Design review of the part built by this model. Coordinates are the model's own, in mm. Coordinates: 2 decimals unless noted, no trailing zeros. Loops run counter-clockwise (first coordinate to the right, second up) from the corner with the lowest first, then second, coordinate; pieces in that order, holes last. Notation, with made-up numbers: M 2,45 L 38,45 A28 ccw 38,78 Z; hole C -27,25.5 d3. An arc over 180 degrees is marked long. Answer as a JSON object with one key per item and string values. Group by question number.
1. Consider section A-A (x = 84.5). State the section outline as (y, z) points, then the cut area to 3 significant figures.
2. Consider section B-B (z = 0.4). Count the separate pieces of the cut face and the enclosed holes in it, then the cut area to 3 significant figures.
3. To check wall thickness, follow probe 1 along X at (y, z) = (-30.5, 0.2); probe 2 along Y at (x, z) = (-32.5, 1.5) (3 decimals); probe 3 along Y at (x, z) = (-54.5, 1.85). State the ranges of each line that lie inside material, in increasing order.
4. Insertion check: pin 1 (0.6 mm diameter, centred on x = -33.5, z = 1, fed in from +Y) (3 decimals). The pin has a flat end and moves straight along its axis. Give the tip position at first contact, or say it passes through.
from build123d import *

# Parameters (mm, degrees)
SKETCH_1_R          = 2.05
SKETCH_1_R_2        = 4
SKETCH_1_R_3        = 2.332988974
SKETCH_1_R_4        = 1.601067765
SKETCH_1_W          = 8.8
SKETCH_1_H          = 2.8
SKETCH_1_W_2        = 2.5
SKETCH_1_H_2        = 8.5
SKETCH_1_W_3        = 8.5
SKETCH_1_H_3        = 2.5
SKETCH_1_W_4        = 241.301375666
SKETCH_1_H_4        = 241.301375666
SKETCH_1_W_5        = 2.3
SKETCH_1_H_5        = 4.3
EXTRUDE_1_DEPTH     = 2
SKETCH_2_W          = 15.371335927
SKETCH_2_H          = 8.514117998
SKETCH_2_W_2        = 8.829080761
SKETCH_2_H_2        = 8.5
SKETCH_2_W_3        = 10.335603127
SKETCH_2_W_4        = 8.5
SKETCH_2_H_3        = 5.29768324
SKETCH_2_H_4        = 6.445558592
SKETCH_2_H_5        = 5.884818728
CUT_EXTRUDE_1_DEPTH = 2
FILLET_1_R          = 2


with BuildPart() as part:
    # 草图1 → 凸台-拉伸1 (new body)
    with BuildSketch(Plane.XY):
        Polygon((-150.650687833, -150.650687833), (-150.650687833, 150.650687833), (150.650687833, 150.650687833), (200.650687833, 150.650687833), (200.650687833, -278.650687833), (150.650687833, -278.650687833), (-150.650687833, -278.650687833), align=None)
        with Locations((0.724285714, -142.895)):
            Circle(SKETCH_1_R, mode=Mode.SUBTRACT)
        with Locations((66.724285714, -142.895)):
            Circle(SKETCH_1_R, mode=Mode.SUBTRACT)
        with Locations((-65.275714286, -142.895)):
            Circle(SKETCH_1_R, mode=Mode.SUBTRACT)
        with Locations((-143.125714286, 66.955)):
            Circle(SKETCH_1_R, mode=Mode.SUBTRACT)
        with Locations((-143.125714286, 0.955)):
            Circle(SKETCH_1_R, mode=Mode.SUBTRACT)
        with Locations((-143.125714286, -65.045)):
            Circle(SKETCH_1_R, mode=Mode.SUBTRACT)
        with Locations((66.874285714, 144.955)):
            Circle(SKETCH_1_R, mode=Mode.SUBTRACT)
        with Locations((0.874285714, 144.955)):
            Circle(SKETCH_1_R, mode=Mode.SUBTRACT)
        with Locations((-65.125714286, 144.955)):
            Circle(SKETCH_1_R, mode=Mode.SUBTRACT)
        with Locations((144.874285714, -65.045)):
            Circle(SKETCH_1_R, mode=Mode.SUBTRACT)
        with Locations((144.874285714, 0.955)):
            Circle(SKETCH_1_R, mode=Mode.SUBTRACT)
        with Locations((144.874285714, 66.955)):
            Circle(SKETCH_1_R, mode=Mode.SUBTRACT)
        with Locations((-130.650687833, -130.650687833)):
            Circle(SKETCH_1_R_2, mode=Mode.SUBTRACT)
        with Locations((-130.650687833, 130.650687833)):
            Circle(SKETCH_1_R_2, mode=Mode.SUBTRACT)
        with Locations((130.650687833, 130.650687833)):
            Circle(SKETCH_1_R_2, mode=Mode.SUBTRACT)
        with Locations((130.650687833, -130.650687833)):
            Circle(SKETCH_1_R_2, mode=Mode.SUBTRACT)
        with Locations((128.234921063, 21.045946403)):
            Circle(SKETCH_1_R_3, mode=Mode.SUBTRACT)
        with Locations((133.709191973, -41.76906745)):
            Circle(SKETCH_1_R_4, mode=Mode.SUBTRACT)
        with Locations((99.724285714, -142.895)):
            Rectangle(SKETCH_1_W, SKETCH_1_H, mode=Mode.SUBTRACT)
        with Locations((33.724285714, -142.895)):
            Rectangle(SKETCH_1_W, SKETCH_1_H, mode=Mode.SUBTRACT)
        with Locations((-32.275714286, -142.895)):
            Rectangle(SKETCH_1_W, SKETCH_1_H, mode=Mode.SUBTRACT)
        with Locations((-98.275714286, -142.895)):
            Rectangle(SKETCH_1_W, SKETCH_1_H, mode=Mode.SUBTRACT)
        with Locations((-143.125714286, 99.955)):
            Rectangle(SKETCH_1_W_2, SKETCH_1_H_2, mode=Mode.SUBTRACT)
        with Locations((-143.125714286, 33.955)):
            Rectangle(SKETCH_1_W_2, SKETCH_1_H_2, mode=Mode.SUBTRACT)
        with Locations((-143.125714286, -32.045)):
            Rectangle(SKETCH_1_W_2, SKETCH_1_H_2, mode=Mode.SUBTRACT)
        with Locations((-143.125714286, -98.045)):
            Rectangle(SKETCH_1_W_2, SKETCH_1_H_2, mode=Mode.SUBTRACT)
        with Locations((99.874285714, 144.955)):
            Rectangle(SKETCH_1_W_3, SKETCH_1_H_3, mode=Mode.SUBTRACT)
        with Locations((33.874285714, 144.955)):
            Rectangle(SKETCH_1_W_3, SKETCH_1_H_3, mode=Mode.SUBTRACT)
        with Locations((-32.125714286, 144.955)):
            Rectangle(SKETCH_1_W_3, SKETCH_1_H_3, mode=Mode.SUBTRACT)
        with Locations((-98.125714286, 144.955)):
            Rectangle(SKETCH_1_W_3, SKETCH_1_H_3, mode=Mode.SUBTRACT)
        with Locations((144.874285714, -98.045)):
            Rectangle(SKETCH_1_W_2, SKETCH_1_H_2, mode=Mode.SUBTRACT)
        with Locations((144.874285714, -32.045)):
            Rectangle(SKETCH_1_W_2, SKETCH_1_H_2, mode=Mode.SUBTRACT)
        with Locations((144.874285714, 33.955)):
            Rectangle(SKETCH_1_W_2, SKETCH_1_H_2, mode=Mode.SUBTRACT)
        with Locations((144.874285714, 99.955)):
            Rectangle(SKETCH_1_W_2, SKETCH_1_H_2, mode=Mode.SUBTRACT)
        Rectangle(SKETCH_1_W_4, SKETCH_1_H_4, mode=Mode.SUBTRACT)
        with Locations((-146.175714286, -272.895)):
            Rectangle(SKETCH_1_W_5, SKETCH_1_H_5, mode=Mode.SUBTRACT)
        with Locations((-146.175714286, -264.895)):
            Rectangle(SKETCH_1_W_5, SKETCH_1_H_5, mode=Mode.SUBTRACT)
        with Locations((-146.175714286, -164.895)):
            Rectangle(SKETCH_1_W_5, SKETCH_1_H_5, mode=Mode.SUBTRACT)
    extrude(amount=EXTRUDE_1_DEPTH)

    # 草图2 → 切除-拉伸1 (cut)
    with BuildSketch(Plane.XY.offset(2)):
        with Locations((-152.06138225, -98.037941001)):
            Rectangle(SKETCH_2_W, SKETCH_2_H)
        with Locations((-148.790254667, -32.045)):
            Rectangle(SKETCH_2_W_2, SKETCH_2_H_2)
        with Locations((-149.54351585, 33.955)):
            Rectangle(SKETCH_2_W_3, SKETCH_2_H_2)
        with Locations((-149.54351585, 99.955)):
            Rectangle(SKETCH_2_W_3, SKETCH_2_H_2)
        with Locations((-98.125714286, 148.85384162)):
            Rectangle(SKETCH_2_W_4, SKETCH_2_H_3)
        with Locations((-32.125714286, 149.427779296)):
            Rectangle(SKETCH_2_W_4, SKETCH_2_H_4)
        with Locations((33.874285714, 149.427779296)):
            Rectangle(SKETCH_2_W_4, SKETCH_2_H_4)
        with Locations((99.874285714, 149.147409364)):
            Rectangle(SKETCH_2_W_4, SKETCH_2_H_5)
    extrude(amount=-CUT_EXTRUDE_1_DEPTH, mode=Mode.SUBTRACT)

    # 圆角1
    fillet_1_edges = [part.edges().sort_by_distance(p)[0] for p in [
        (-150.650687833, -102.295, 1),
        (-150.650687833, -93.780882002, 1),
        (-150.650687833, -36.295, 1),
        (-150.650687833, -27.795, 1),
        (-150.650687833, 29.705, 1),
        (-150.650687833, 38.205, 1),
        (-150.650687833, 95.705, 1),
        (-150.650687833, 104.205, 1),
        (-102.375714286, 150.650687833, 1),
        (-93.875714286, 150.650687833, 1),
        (-36.375714286, 150.650687833, 1),
        (-27.875714286, 150.650687833, 1),
        (29.624285714, 150.650687833, 1),
        (38.124285714, 150.650687833, 1),
        (95.624285714, 150.650687833, 1),
        (104.124285714, 150.650687833, 1),
    ]]
    fillet(fillet_1_edges, radius=FILLET_1_R)


solid = part.part
Findings below:
{
 "1": {"outline": "M -278.65,0 L -120.65,0 L -120.65,2 L -278.65,2 Z; M 120.65,0 L 150.65,0 L 150.65,2 L 120.65,2 Z", "area": "376 mm^2"},
 "2": {"separate pieces": "1", "enclosed holes": "30", "area": "91,400 mm^2"},
 "3": {"probe 1": "x = -141.88 to -120.65, 120.65 to 143.62, 146.12 to 200.65", "probe 2": "y = -278.651 to -144.295, -141.495 to -120.651, 120.651 to 143.705", "probe 3": "y = -278.65 to -120.65, 120.65 to 150.65"},
 "4": {"pin 1": "stops at y = 143.705"}
}
